Design review of the part shown in the three views and the two pictorial views. Dimensions are in mm from the part's minimum x, y and z. A direction names the side the tool comes from. Give positions to 0.01 mm unless a question says otherwise; leave off trailing zeros. Order: outer loops, then holes, each group sorted by start corner. A loop starts at its lowest first (then second) coordinate and runs counter-clockwise, first axis right, second up. Notation, with made-up numbers: M -29,73 L -20,73 A26 cw -20,100 Z; hole C -17,71 d11. An arc over 180 degrees is marked long. Answer as a JSON object with one key per item and string values.
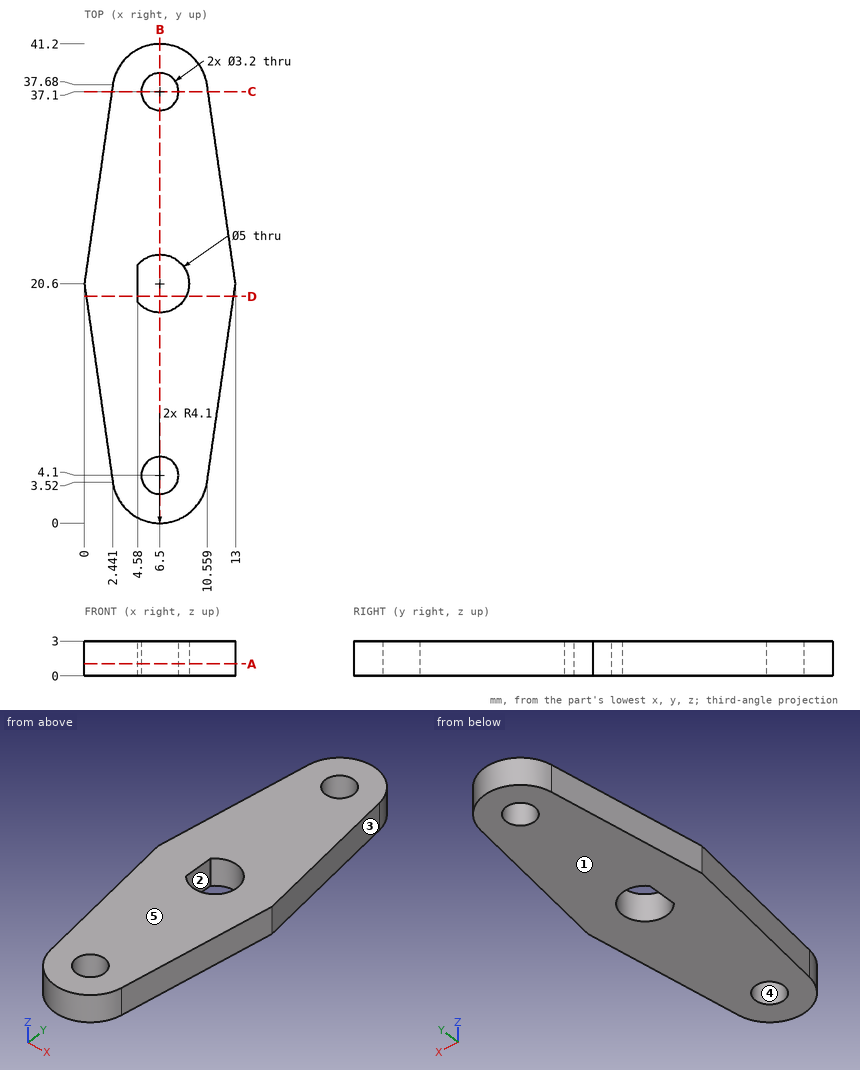
(1) Insertion check: pin 1 (6.5 mm diameter, centred on x = 6.5, y = 20.6, fed in from +Z); pin 2 (1.5 mm diameter, centred on x = 4, z = 2.5, fed in from +Y). Each pin has a flat end and moves straight along its axis. Give the tip position at first contact, or say it passes through.
Checked values:
{"pin 1": "stops at z = 3", "pin 2": "stops at y = 40.81"}
(2) Draft analysis for pull direction Y (two halves, no side actions). For the marked faces 3, 4 and 5, state which applies: +Y half, -Y half, draft (parallel to the pull), parting line (faces both ways), or undercut.
Checked values:
{"face 3": "+Y half", "face 4": "undercut", "face 5": "draft"}
(3) We need section D-D (y = 19.5). Write out the cut boundary in (x, z) (1 decimal).
Checked values:
{"outline": "M 0.2,0 L 4.6,0 L 4.6,3 L 0.2,3 Z; M 8.7,0 L 12.8,0 L 12.8,3 L 8.7,3 Z"}
(4) We need section B-B (x = 6.5). Write out the cut boundary in (y, z).
Checked values:
{"outline": "M 0,0 L 2.5,0 L 2.5,3 L 0,3 Z; M 5.7,0 L 18.1,0 L 18.1,3 L 5.7,3 Z; M 23.1,0 L 35.5,0 L 35.5,3 L 23.1,3 Z; M 38.7,0 L 41.2,0 L 41.2,3 L 38.7,3 Z"}
(5) We need section A-A (z = 1.05). Write out the cut boundary in (x, y), plus the area to 3 significant figures.
Checked values:
{"outline": "M 0,20.6 L 2.44,3.52 A4.1 ccw 10.56,3.52 L 13,20.6 L 10.56,37.68 A4.1 ccw 2.44,37.68 Z; hole M 4.58,19 A2.5 ccw long 4.58,22.2 Z; hole C 6.5,4.1 d3.2; hole C 6.5,37.1 d3.2", "area": "370 mm^2"}
(6) Tool access review of the marked faces 1 and 2: name each direction out of +Z, -Z, +X, -X, +Y, -Y from which nothing blocks a thin tool from reaching the whole face with its end or side.
Checked values:
{"face 1": "-Z, +X, -X, +Y, -Y", "face 2": "+Z, -Z"}
(7) To check wall thickness, follow L1, parallel to Y at x = 7.75, z = 2.7 (1 decimal); L2, parallel to X at y = 20.6, z = 1.2; L3, parallel to Y at x = 8.5, z = 2.4. State the ranges of each line that lie inside material, in increasing order. Write a range as from..to.
Checked values:
{"L1": "y = 0.2..3.1, 5.1..18.4, 22.8..36.1, 38.1..41", "L2": "x = 0..4.58, 9..13", "L3": "y = 0.52..19.1, 22.1..40.68"}
(8) We need section C-C (y = 37.1). Write out the cut boundary in (x, z).
Checked values:
{"outline": "M 2.36,0 L 4.9,0 L 4.9,3 L 2.36,3 Z; M 8.1,0 L 10.64,0 L 10.64,3 L 8.1,3 Z"}
